Verification items for the finished model (mm, model axes). A direction names the side the tool comes from. Coordinates: 2 decimals unless noted, no trailing zeros. Return JSON: item names as keys, results as strings. Group by question number.
1. Gauge pin test, flat ends, axial feed: pin 1 (10 mm diameter, centred on x = -284, y = 104.5, fed in from -Z); pin 2 (1.6 mm diameter, centred on y = 86.66, z = 2.5, fed in from +X); pin 3 (4 mm diameter, centred on x = -278.5, y = 97.5, fed in from +Z); pin 4 (1.5 mm diameter, centred on y = 123.5, z = 5, fed in from -X). Record the tip position at first contact, or that the pin passes through.
2. Material ranges on line 1 along Z through (x, y) = (-258, 129.5); line 2 along X through (y, z) = (122.5, 5.25); line 3 along Y through (x, z) = (-270.5, 2.25), recorded low to high.
3. Mould release check, pull along X, two halves, no side actions. Record for faces 6 (the flat face through (-296.717, 105.537, 3.24)), 7 (the cylindrical face through (-289.24, 118.42, 4.62)), 8 (the cylindrical face through (-284.29, 89.29, 3.94)): +X half, -X half, draft (parallel to the pull), parting line (faces both ways), or undercut.
4. Set-up check for faces 1 (the flat face through (-283.204, 132.09, 3.854)), 2 (the flat face through (-271.817, 87, 4)), 3 (the flat face through (-295.536, 110.305, 5.591)), 4 (the flat face through (-259, 86.656, 4)), 5 (the flat face through (-261.817, 86, 1)): record each of +Z, -Z, +X, -X, +Y, -Y from which the full face is reachable in a straight line by a thin tool's end or side.
```python
from build123d import *

# Parameters (mm, degrees)
EXTRUDE_1_DEPTH          = 5
SKETCH_5_W               = 5
SKETCH_5_H               = 50
SKETCH_2_W               = 20
SKETCH_2_H               = 5
CUT_EXTRUDE_2_DEPTH      = 698.009362047
CUT_EXTRUDE_2_DEPTH_BACK = 698.009362047
SKETCH_8_R               = 2
SKETCH_12_R              = 6
SKETCH_12_R_2            = 2
CUT_EXTRUDE_6_DEPTH      = 346.897812083
CUT_EXTRUDE_7_DEPTH      = 346.897812083
CUT_EXTRUDE_7_DEPTH_BACK = 346.897812083
SKETCH_13_R              = 2
SKETCH_11_R              = 6
CUT_EXTRUDE_5_DEPTH      = 692.343248918
SCALE_1_SCALE            = 0.5


with BuildPart() as part:
    # 草图1 → 凸台-拉伸1 (new body)
    with BuildSketch(Plane.XY.offset(5)):
        with BuildLine():
            Line((-531.259329651, 335.424320593), (-597.842921786, 202.257136323))
            ThreePointArc((-597.842921786, 202.257136323), (-596.967394134, 182.798242171), (-579.954377966, 173.312864413))
            Line((-579.954377966, 173.312864413), (-512.315057741, 173.312864413))
            Line((-512.315057741, 173.312864413), (-512.315057741, 330.952184638))
            ThreePointArc((-512.315057741, 330.952184638), (-520.017528536, 340.684674533), (-531.259329651, 335.424320593))
        make_face()
    extrude(amount=EXTRUDE_1_DEPTH)

    # 草图5 → 旋转1 (revolve)
    with BuildSketch(Plane(origin=(-559.177191958, 279.588595979, 0), x_dir=(0, 0, 1), z_dir=(-0.894427190999916, 0.4472135954999578, 0))):
        with Locations((7.5, -42.016481195)):
            Rectangle(SKETCH_5_W, SKETCH_5_H)
    revolve(axis=Axis((-566.787193696, 264.368592503, 10), (-0.4472135954999577, -0.894427190999916, 0)))

    # 草图2 → 旋转2 (revolve)
    with BuildSketch(Plane.XZ.offset(-173.312864413)):
        with Locations((-533.634717854, 7.5)):
            Rectangle(SKETCH_2_W, SKETCH_2_H)
    revolve(axis=Axis((-543.634717854, 173.312864413, 5), (1, 0, 0)))

    # 草图8 → 切除-拉伸2 (cut, two sides: drawn at the far end of the back side and taken through both)
    with BuildSketch(Plane(origin=(-29.970681513, -59.941363026, 0), x_dir=(0.894427190999916, -0.4472135954999577, 0), z_dir=(-0.4472135954999577, -0.894427190999916, 0)).offset(-CUT_EXTRUDE_2_DEPTH_BACK)):
        with Locations((-625.179106343, 10)):
            Circle(SKETCH_8_R)
    extrude(amount=CUT_EXTRUDE_2_DEPTH + CUT_EXTRUDE_2_DEPTH_BACK, mode=Mode.SUBTRACT)

    # 草图12 → 切除-拉伸6 (cut, through all)
    with BuildSketch(Plane.ZY.offset(543.634717854)):
        with Locations((5, 173.312864413)):
            Circle(SKETCH_12_R)
        with Locations((5, 173.312864413)):
            Circle(SKETCH_12_R_2, mode=Mode.SUBTRACT)
    extrude(amount=CUT_EXTRUDE_6_DEPTH, mode=Mode.SUBTRACT)

    # 草图13 → 切除-拉伸7 (cut, two sides: drawn at the far end of the back side and taken through both)
    with BuildSketch(Plane.ZY.offset(543.634717854).offset(-CUT_EXTRUDE_7_DEPTH_BACK)):
        with Locations((5, 173.312864413)):
            Circle(SKETCH_13_R)
    extrude(amount=CUT_EXTRUDE_7_DEPTH + CUT_EXTRUDE_7_DEPTH_BACK, mode=Mode.SUBTRACT)

    # 草图11 → 切除-拉伸5 (cut, through all)
    with BuildSketch(Plane(origin=(-7.610001738, -15.220003476, 0), x_dir=(0.8944271909999161, -0.4472135954999577, 0), z_dir=(0.4472135954999577, 0.8944271909999161, 0))):
        with Locations((-625.179106343, -10)):
            Circle(SKETCH_11_R)
    extrude(amount=CUT_EXTRUDE_5_DEPTH, mode=Mode.SUBTRACT)


with BuildPart() as part_1:
    # 缩放比例1: scaled about (0, 0, 0)
    add(part.part.scale(SCALE_1_SCALE))


solid = part_1.part
```
Answers follow:
{
 "1": {"pin 1": "z = 2.5", "pin 2": "through", "pin 3": "z = 5", "pin 4": "x = -290.91"},
 "2": {"line 1": "2.5 to 5", "line 2": "-291.02 to -289.32, -287.15 to -285.45", "line 3": "84.17 to 85.69, 87.62 to 89.14"},
 "3": {"face 6": "-X half", "face 7": "undercut", "face 8": "draft"},
 "4": {"face 1": "+Z, +Y", "face 2": "-Z, -X, -Y", "face 3": "+Z, -X", "face 4": "+Z, -Z, +X, -Y", "face 5": "-Z, +X, -Y"}
}
